Geometry check sheet. Reference: the model listing, model coordinates, mm. Face numbers are marked on the shaded views. A direction names the side the tool comes from. Give positions to 0.01 mm unless a question says otherwise; leave off trailing zeros. Order: outer loops, then holes, each group sorted by start corner. A loop starts at its lowest first (then second) coordinate and runs counter-clockwise, first axis right, second up. Notation, with made-up numbers: M 10,33 L 14,33 A22 ccw 14,68 Z; hole C 25,47 d11. An arc over 180 degrees is marked long. Put each result on its own line as item: value. Start each with the question number.
Q1. Mould release check, pull along Y, two halves, no side actions. Record for the marked faces 1, 2 and 3: +Y half, -Y half, draft (parallel to the pull), parting line (faces both ways), or undercut.
Q2. Section check D-D on x = -15. Record the cut outline in (y, z), then the cut area to 3 significant figures.
Q3. Section check A-A on x = 39. Record the cut outline in (y, z), then the cut area to 3 significant figures.
Q4. Material ranges on L1, parallel to Y at x = 0, z = 17.5; L2, parallel to Y at x = -11, z = 15.5; L3, parallel to X at y = 0.5, z = 16, recorded low to high.
Q5. Section check C-C on z = 21. Record the cut outline in (x, y), then the cut area to 3 significant figures.
Q6. Section check B-B on y = -22. Record the cut outline in (x, z).
Q7. Go/stop test with flat-tipped pins: pin 1 (6 mm diameter, centred on x = 19, z = 20.5, fed in from +Y); pin 2 (8 mm diameter, centred on y = 1.5, z = 9.5, fed in from -X); pin 3 (1.5 mm diameter, centred on x = 35, z = 18.5, fed in from +Y); pin 4 (5.5 mm diameter, centred on x = 2, z = 8, fed in from +Y). Record where each tip stops, or that it passes through.
Q8. Access from +Z, -Z, +X, -X, +Y, -Y to the whole of each face (thin tool, end or side, straight path). Record for the marked faces 4, 5 and 6.
```python
from build123d import *

# Parameters (mm, degrees)
F1_DEPTH = 27.686


with BuildPart() as f1:
    # F0 (on Top) → F1 (new body)
    with BuildSketch(Plane.XY):
        with BuildLine():
            ThreePointArc((-7.984679, -18.871297), (-11.319605, 17.080618), (20.490997, 0))
            ThreePointArc((20.490997, 0), (17.080618, -11.319605), (7.984679, -18.871297))
            Line((7.984679, -18.871297), (14.139757, -18.871297))
            ThreePointArc((14.139757, -18.871297), (16.449072, -16.896349), (18.485251, -14.640837))
            ThreePointArc((18.485251, -14.640837), (22.270579, -7.751124), (23.580895, 0))
            ThreePointArc((23.580895, 0), (-7.751124, 22.270579), (-18.485251, -14.640837))
            ThreePointArc((-18.485251, -14.640837), (-16.449072, -16.896349), (-14.139757, -18.871297))
            Line((-14.139757, -18.871297), (-7.984679, -18.871297))
        make_face()
        with BuildLine():
            Line((-40.005073, -18.871297), (-14.139757, -18.871297))
            ThreePointArc((-14.139757, -18.871297), (-16.449072, -16.896349), (-18.485251, -14.640837))
            Line((-18.485251, -14.640837), (-42.802565, -14.640837))
            Line((-42.802565, -14.640837), (-42.802565, -72.456613))
            Line((-42.802565, -72.456613), (-23.49944, -72.456613))
            Line((-23.49944, -72.456613), (-23.49944, -67.421012))
            Line((-23.49944, -67.421012), (-40.005073, -67.421012))
            Line((-40.005073, -67.421012), (-40.005073, -18.871297))
        make_face()
        with BuildLine():
            ThreePointArc((18.485251, -14.640837), (16.449072, -16.896349), (14.139757, -18.871297))
            Line((14.139757, -18.871297), (41.683532, -18.871297))
            Line((41.683532, -18.871297), (41.683532, -67.421012))
            Line((41.683532, -67.421012), (26.762667, -67.421012))
            Line((26.762667, -67.421012), (26.762667, -72.456613))
            Line((26.762667, -72.456613), (45.320351, -72.456613))
            Line((45.320351, -72.456613), (45.320351, -14.640837))
            Line((45.320351, -14.640837), (18.485251, -14.640837))
        make_face()
        Polygon((-20.142378, -67.421012), (-23.49944, -67.421012), (-23.49944, -72.456613), (-2.309161, -72.456613), (-5.808478, -67.421012), (-8.672413, -67.421012), align=None)
        Polygon((26.762667, -72.456613), (26.762667, -67.421012), (22.93993, -67.421012), (10.350944, -67.421012), (5.582281, -67.421012), (1.503095, -72.456613), (5.31535, -72.456613), align=None)
        Polygon((-5.808478, -67.421012), (-2.309161, -72.456613), (1.503095, -72.456613), (5.582281, -67.421012), align=None)
        Polygon((22.93993, -67.421012), (26.762667, -67.421012), (26.762667, -41.274629), (24.61846, -43.921571), (5.582281, -67.421012), (10.350944, -67.421012), (22.93993, -50.915454), align=None)
        Polygon((-23.49944, -41.963287), (-23.49944, -67.421012), (-20.142378, -67.421012), (-20.142378, -50.915454), (-8.672413, -67.421012), (-5.808478, -67.421012), align=None)
    extrude(amount=F1_DEPTH)


solid = f1.part
```
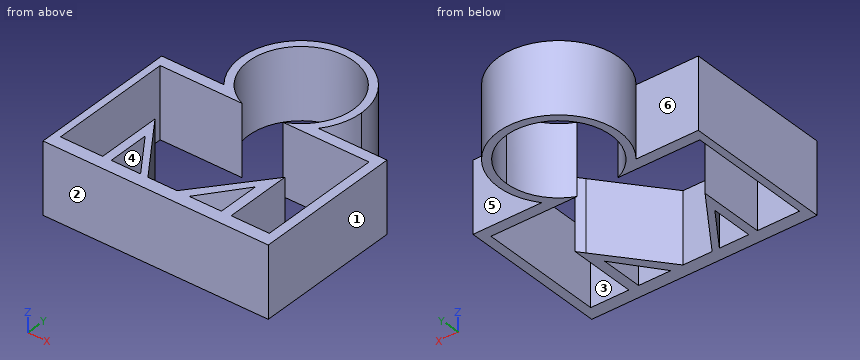
Results found:
1. face 1: draft
1. face 2: -Y half
1. face 3: undercut
2. outline: M -72.46,0 L -67.42,0 L -67.42,27.69 L -72.46,27.69 Z; M -58.32,0 L -54.19,0 L -54.19,27.69 L -58.32,27.69 Z; M -18.87,0 L -13.96,0 L -13.96,27.69 L -18.87,27.69 Z; M 13.96,0 L 18.2,0 L 18.2,27.69 L 13.96,27.69 Z
2. area: 507 mm^2
3. outline: M -72.46,0 L -67.42,0 L -67.42,27.69 L -72.46,27.69 Z; M -18.87,0 L -14.64,0 L -14.64,27.69 L -18.87,27.69 Z
3. area: 257 mm^2
4. L1: y = -72.46 to -67.42, 20.49 to 23.58
4. L2: y = -72.46 to -67.42, -64.07 to -59.95, -18.87 to -17.29, 17.29 to 20.86
4. L3: x = -23.58 to -20.48, 20.48 to 23.58
5. outline: M -42.8,-72.46 L 45.32,-72.46 L 45.32,-14.64 L 18.49,-14.64 A23.58 ccw long -18.49,-14.64 L -42.8,-14.64 Z; hole M -40.01,-67.42 L -23.5,-67.42 L -23.5,-41.96 L -5.81,-67.42 L 5.58,-67.42 L 26.76,-41.27 L 26.76,-67.42 L 41.68,-67.42 L 41.68,-18.87 L 7.98,-18.87 A20.49 ccw 20.49,0 A20.49 ccw long -7.98,-18.87 L -40.01,-18.87 Z; hole M -20.14,-67.42 L -8.67,-67.42 L -20.14,-50.92 Z; hole M 10.35,-67.42 L 22.94,-67.42 L 22.94,-50.92 Z
5. area: 1,650 mm^2
6. outline: M -42.8,0 L -40.01,0 L -40.01,27.69 L -42.8,27.69 Z; M 41.68,0 L 45.32,0 L 45.32,27.69 L 41.68,27.69 Z
7. pin 1: stops at y = 17.32
7. pin 2: stops at x = -23.58
7. pin 3: stops at y = -14.64
7. pin 4: stops at y = 23.58
8. face 4: +Z, -Z
8. face 5: +Z, -Z, +X
8. face 6: +Z, -Z, -X
